Source: three-view drawing plus pictorial views. Frame: mm from the lowest corner of the part. Coordinates: 2 decimals unless noted, no trailing zeros. Write each loop counter-clockwise with the first axis right and the second up, starting at its lowest first coordinate (ties: lowest second). Pieces come first, ordered by that corner, then holes. Notation, with made-up numbers: M -13,-19.75 L 19,-19.75 A31 ccw 19,19.25 Z; hole C -34,-29.75 d3. An arc over 180 degrees is marked long. Write item = value, one per line. Start each with the question number.
Item 1: Section D-D on y = 6. Output: boundary loops of the cut face in (x, z), plus the area to 3 significant figures.
Item 2: Pull-direction query (Z, two-part tool) for the marked faces 1, 2 and 3; classes: +Z half, -Z half, draft (parallel to the pull), parting line (faces both ways), or undercut.
Item 3: Ray query, L1, parallel to X at y = 6.5, z = 6; L2, parallel to X at y = 7.5, z = 7; L3, parallel to Z at x = 18.5, y = 5.75. Return the intervals inside material, ascending. Write a range as [from, to].
Item 4: Section B-B on z = 6. Output: boundary loops of the cut face in (x, y), plus the area to 3 significant figures.
Item 5: First-contact query: pin 1 Ø6 at (x, z) = (17.5, 5.5) entering from +Y; pin 2 Ø2 at (x, z) = (8, 7.5) entering from -Y. Flat tips, straight axial feed; report the tip coordinate or a pass-through.
Item 6: Section C-C on y = 3. Output: boundary loops of the cut face in (x, z), plus the area to 3 significant figures.
Item 7: Section A-A on x = 18.5. Output: boundary loops of the cut face in (y, z).
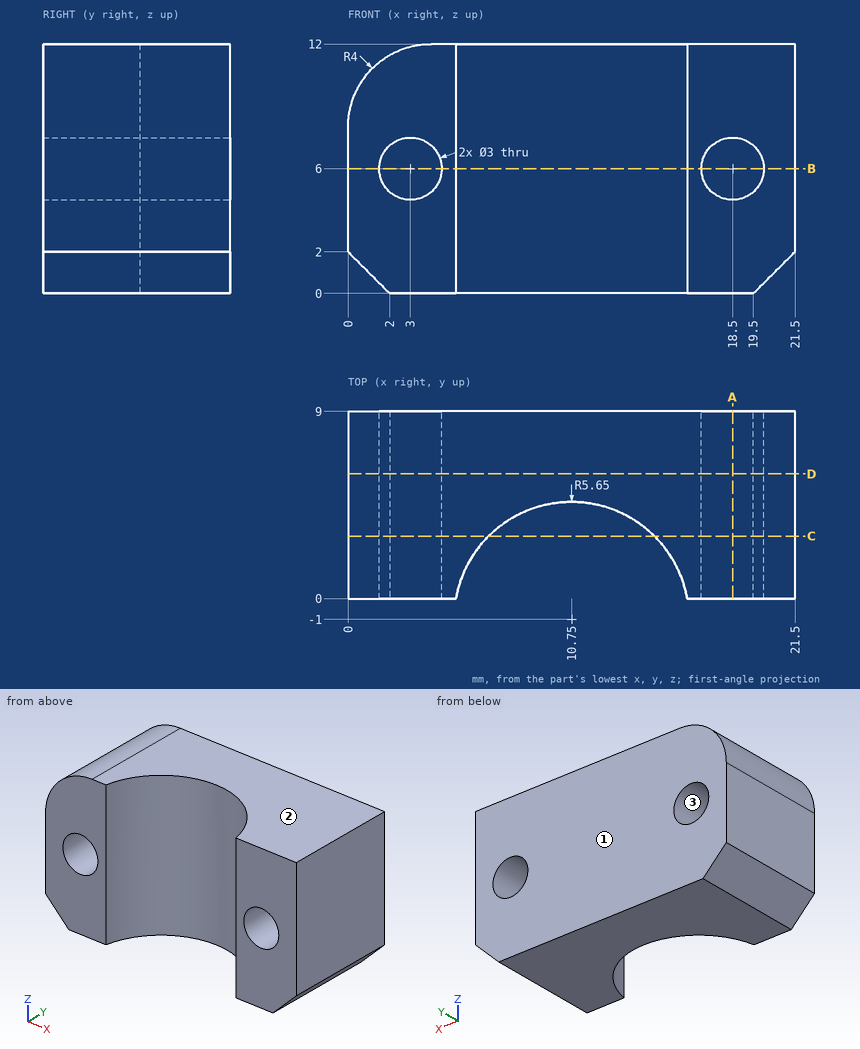
Responses:
q1.outline = M 0,2 L 2,0 L 19.5,0 L 21.5,2 L 21.5,12 L 4,12 A4 ccw 0,8 Z; hole C 3,6 d3; hole C 18.5,6 d3
q1.area = 236 mm²
q2.face_1 = draft
q2.face_2 = +Z half
q2.face_3 = undercut
q3.L1 = [0, 1.5], [4.5, 17], [20, 21.5]
q3.L2 = [0, 1.88], [4.12, 17.38], [19.62, 21.5]
q3.L3 = [0, 4.5], [7.5, 12]
q4.outline = M 0,0 L 1.5,0 L 1.5,9 L 0,9 Z; M 4.5,0 L 5.19,0 A5.65 cw 16.31,0 L 17,0 L 17,9 L 4.5,9 Z; M 20,0 L 21.5,0 L 21.5,9 L 20,9 Z
q4.area = 101 mm²
q5.pin_1 = 9
q5.pin_2 = 3.23
q6.outline = M 0,2 L 2,0 L 6.76,0 L 6.76,12 L 4,12 A4 ccw 0,8 Z; M 14.74,0 L 19.5,0 L 21.5,2 L 21.5,12 L 14.74,12 Z; hole C 3,6 d3; hole C 18.5,6 d3
q6.area = 141 mm²
q7.outline = M 0,0 L 9,0 L 9,4.5 L 0,4.5 Z; M 0,7.5 L 9,7.5 L 9,12 L 0,12 Z
